```python
from build123d import *

# Parameters (mm, degrees)
F1_DEPTH = 4.7625
F8_DEPTH = 25.4
F9_R     = 1.27


with BuildPart() as f1:
    # F0 (on Top) → F1 (new body, symmetric)
    with BuildSketch(Plane.XY):
        with BuildLine():
            Line((0, 44.45), (0, 0))
            Line((0, 0), (50.8, 0))
            ThreePointArc((50.8, 0), (68.7605122421, 7.4394877579), (76.2, 25.4))
            Line((76.2, 25.4), (76.2, 44.45))
            Line((76.2, 44.45), (0, 44.45))
        make_face()
    extrude(amount=F1_DEPTH, both=True)


with BuildPart() as f4:
    # F4: sweep along a path in F3
    with BuildLine(Plane.XY.offset(4.7625)) as f4_path:
        Line((0, 0), (50.8, 0))
        ThreePointArc((50.8, 0), (68.7605122421, 7.4394877579), (76.2, 25.4))
        Line((76.2, 25.4), (76.2, 44.45))
    # F2 (on face) → F4 (sweep)
    with BuildSketch(Plane(origin=(0, 0, 0), x_dir=(0, -1, 0), z_dir=(-1, 0, 0))):
        with BuildLine():
            Line((0, 4.7625), (-19.05, 4.7625))
            ThreePointArc((-19.05, 4.7625), (-13.4517306294, 2.3955307002), (-7.4275916867, 1.5875))
            Line((-7.4275916867, 1.5875), (0, 1.5875))
            Line((0, 1.5875), (0, 4.7625))
        make_face()
    sweep(path=f4_path.line)


with BuildPart() as f5_1:
    # F5: instance of F4
    add(f4.part.mirror(Plane.XY))


with BuildPart() as f1_1:
    add(f1.part)

    # F6: cut F4, F5_1
    add(f4.part, mode=Mode.SUBTRACT)
    add(f5_1.part, mode=Mode.SUBTRACT)

    # F7 (on face) → F8 (cut)
    with BuildSketch(Plane(origin=(0, 0, 0), x_dir=(0, -1, 0), z_dir=(-1, 0, 0))):
        with BuildLine():
            Line((-38.1, -3.175), (-25.4, -3.175))
            ThreePointArc((-25.4, -3.175), (-23.1549359697, -2.2450640303), (-22.225, 0))
            ThreePointArc((-22.225, 0), (-23.1549359697, 2.2450640303), (-25.4, 3.175))
            Line((-25.4, 3.175), (-38.1, 3.175))
            ThreePointArc((-38.1, 3.175), (-40.3450640303, 2.2450640303), (-41.275, 0))
            ThreePointArc((-41.275, 0), (-40.3450640303, -2.2450640303), (-38.1, -3.175))
        make_face()
    extrude(amount=-F8_DEPTH, mode=Mode.SUBTRACT)

    # F9
    f9_edges = [f1_1.edges().sort_by_distance(p)[0] for p in [
        (28.575, 44.45, 4.7625),
        (28.575, 44.45, -4.7625),
        (25.4, 0, 1.5875),
        (68.760512, 7.439488, 1.5875),
        (76.2, 34.925, 1.5875),
        (25.4, 0, -1.5875),
        (68.760512, 7.439488, -1.5875),
        (76.2, 34.925, -1.5875),
    ]]
    fillet(f9_edges, radius=F9_R)


solid = f1_1.part
```
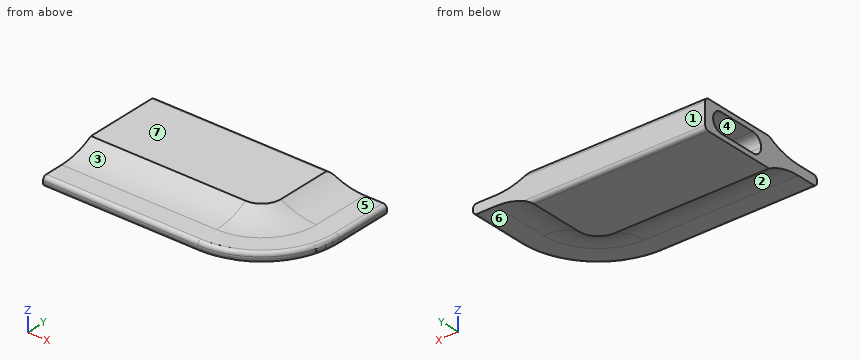
Build history of the part. All positions in model axes, mm. Face numbers are marked on the shaded views. A direction names the side the tool comes from. Give positions to 0.01 mm unless a question says otherwise; leave off trailing zeros. Order: outer loops, then holes, each group sorted by start corner. A loop starts at its lowest first (then second) coordinate and runs counter-clockwise, first axis right, second up. Notation, with made-up numbers: M 2.5,-22 L 61.5,-22 A14 cw 61.5,-12 Z; hole C -34,12 d4. An arc over 180 degrees is marked long. Return JSON: item names as keys, results as strings.
Q1. Band-saw the part on C-C (x = 31). Give the cut face in (y, z), then the cut area to 3 significant figures.
Answer list:
{"outline": "M 0,-0.32 A1.27 ccw 1.27,-1.59 L 7.43,-1.59 A22.86 cw 19.05,-4.76 L 43.18,-4.76 A1.27 ccw 44.45,-3.49 L 44.45,3.49 A1.27 ccw 43.18,4.76 L 19.05,4.76 A22.86 cw 7.43,1.59 L 1.27,1.59 A1.27 ccw 0,0.32 Z", "area": "325 mm^2"}
Q2. Flat gauge pins, fed straight in: pin 1 (3 mm diameter, centred on y = 29.5, z = -1.5, fed in from -X); pin 2 (1.5 mm diameter, centred on x = 53.5, z = -2, fed in from -Y); pin 3 (2 mm diameter, centred on y = 5.5, z = -0.5, fed in from -X). Where does each tip first touch, or does it go through?
Answer list:
{"pin 1": "stops at x = 25.4", "pin 2": "stops at y = 0.55", "pin 3": "stops at x = 0"}
Q3. 3-axis set-ups, long thin cutter, end or side, ignore diameter. For the marked faces 5, 6 and 7: which of +Z, -Z, +X, -X, +Y, -Y reach the whole face in a straight line?
Answer list:
{"face 5": "+Z, +X, -Y", "face 6": "-Z, +X, -Y", "face 7": "+Z, +X, -X, +Y, -Y"}
Q4. Two-plate mould, pull along Z, no slides. Class the marked faces 1, 2, 3 and 4: pulls with the +Z half, pulls with the -Z half, needs draft (parallel to the pull), parting line crosses it, or undercut.
Answer list:
{"face 1": "needs draft", "face 2": "pulls with the -Z half", "face 3": "pulls with the +Z half", "face 4": "undercut"}
Q5. Wall check: probe 1 along Z at (x, y) = (16, 27.5) (1 decimal); probe 2 along Y at (x, z) = (5, -0.25); probe 3 along Y at (x, z) = (31, 0.5). Give the ranges that are in metal, low to high. Write a range as from..to.
Answer list:
{"probe 1": "z = -4.8..-3.2, 3.2..4.8", "probe 2": "y = 0..22.23, 41.27..44.45", "probe 3": "y = 0.01..44.45"}
